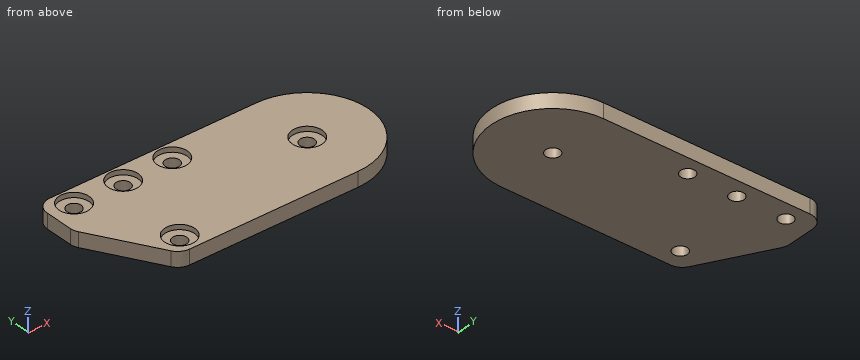
```python
from build123d import *

# Parameters (mm, degrees)
SKETCH_2_R          = 1.45
EXTRUDE_1_DEPTH     = 3
SKETCH_3_R          = 1.45
EXTRUDE_2_DEPTH     = 3
SKETCH_5_R          = 3.05
CUT_EXTRUDE_1_DEPTH = 1
EXTRUDE_3_DEPTH     = 3
SKETCH_7_R          = 3.05
CUT_EXTRUDE_4_DEPTH = 1
FILLET_1_R          = 3
SKETCH_10_R         = 3.05
CUT_EXTRUDE_6_DEPTH = 1


with BuildPart() as part:
    # 草图2 → 凸台-拉伸1 (new body)
    with BuildSketch(Plane.XY):
        with BuildLine():
            Line((-10, -7), (-10, -16.423561614))
            Line((-10, -16.423561614), (30.724748208, -31.24615776))
            ThreePointArc((30.724748208, -31.24615776), (47.310096913, -21.670602221), (35, -7))
            Line((35, -7), (-10, -7))
        make_face()
        with Locations((35, -19.5)):
            Circle(SKETCH_2_R, mode=Mode.SUBTRACT)
        with Locations((15, -10.5)):
            Circle(SKETCH_2_R, mode=Mode.SUBTRACT)
        with Locations((5, -10.5)):
            Circle(SKETCH_2_R, mode=Mode.SUBTRACT)
        with Locations((-5, -10.5)):
            Circle(SKETCH_2_R, mode=Mode.SUBTRACT)
    extrude(amount=EXTRUDE_1_DEPTH)

    # 草图3 → 凸台-拉伸2 (add)
    with BuildSketch(Plane.XY.offset(3)):
        Polygon((-10, -16.423561614), (32.795912741, -32), (-1.006939105, -32), align=None)
        with Locations((2, -28)):
            Circle(SKETCH_3_R, mode=Mode.SUBTRACT)
    extrude(amount=-EXTRUDE_2_DEPTH)

    # 草图5 → 切除-拉伸1 (cut)
    with BuildSketch(Plane.XY.offset(3)):
        with Locations((-5, -10.5)):
            Circle(SKETCH_5_R)
        with Locations((5, -10.5)):
            Circle(SKETCH_5_R)
        with Locations((15, -10.5)):
            Circle(SKETCH_5_R)
    extrude(amount=-CUT_EXTRUDE_1_DEPTH, mode=Mode.SUBTRACT)

    # 草图8 → 凸台-拉伸3 (add)
    with BuildSketch(Plane.XY.offset(3)):
        Polygon((32.795912741, -32), (35, -32), (30.724748208, -31.24615776), align=None)
    extrude(amount=-EXTRUDE_3_DEPTH)

    # 草图7 → 切除-拉伸4 (cut)
    with BuildSketch(Plane.XY.offset(3)):
        with Locations((2, -28)):
            Circle(SKETCH_7_R)
    extrude(amount=-CUT_EXTRUDE_4_DEPTH, mode=Mode.SUBTRACT)

    # 圆角1
    fillet_1_edges = [part.edges().sort_by_distance(p)[0] for p in [
        (-1.006939105, -32, 1.5),
        (-10, -16.423561614, 1.5),
        (-10, -7, 1.5),
    ]]
    fillet(fillet_1_edges, radius=FILLET_1_R)

    # 草图10 → 切除-拉伸6 (cut)
    with BuildSketch(Plane.XY.offset(3)):
        with Locations((35, -19.5)):
            Circle(SKETCH_10_R)
    extrude(amount=-CUT_EXTRUDE_6_DEPTH, mode=Mode.SUBTRACT)


solid = part.part
```
Read the model definition and answer for the solid it produces. Units are mm, in the model's axes. Coordinates: 2 decimals unless noted, no trailing zeros. Write each loop counter-clockwise with the first axis right and the second up, starting at its lowest first coordinate (ties: lowest second). Pieces come first, ordered by that corner, then holes. Notation, with made-up numbers: (77.5, 42.25) -> (102.5, 42.25) arc R31 cw to (102.5, 80.25) -> close; hole circle Ø1 at (45.5, 57). An arc over 180 degrees is marked (long way). Answer as a JSON object with one key per item and string values.
Q1. The part is cut by section A-A on x = 15. Give the vertices of the cut face in (y, z), then the cut area to 3 significant figures.
The answers:
{"outline": "(-32, 0) -> (-11.95, 0) -> (-11.95, 2) -> (-13.55, 2) -> (-13.55, 3) -> (-32, 3) -> close; (-9.05, 0) -> (-7, 0) -> (-7, 3) -> (-7.45, 3) -> (-7.45, 2) -> (-9.05, 2) -> close", "area": "63.1 mm2"}
Q2. The part is cut by section B-B on z = 1.15. Give the vertices of the cut face in (x, y).
The answers:
{"outline": "(-10, -15.62) arc R3 ccw to (-9.6, -17.12) -> (-1.87, -30.5) arc R3 ccw to (0.73, -32) -> (35, -32) arc R12.5 ccw to (35, -7) -> (-7, -7) arc R3 ccw to (-10, -10) -> close; hole circle Ø2.9 at (-5, -10.5); hole circle Ø2.9 at (2, -28); hole circle Ø2.9 at (5, -10.5); hole circle Ø2.9 at (15, -10.5); hole circle Ø2.9 at (35, -19.5)"}
Q3. Consider line 1 (Y direction, x = 35, z = 2.7); line 2 (Y direction, x = 35, z = 0.95); line 3 (X direction, y = -10, z = 1). Determine where each line is inside the solid, lowest interval first. Write a range as [from, to].
The answers:
{"line 1": "y = [-32, -22.55], [-16.45, -7]", "line 2": "y = [-32, -20.95], [-18.05, -7]", "line 3": "x = [-10, -6.36], [-3.64, 3.64], [6.36, 13.64], [16.36, 43.12]"}
Q4. Flat-ended cylindrical pins translate along their axes: pin 1 Ø1.8 at (x, y) = (-6, -10.5) entering from +Z; pin 2 Ø3.5 at (x, y) = (15, -10.5) entering from -Z; pin 3 Ø2.5 at (x, y) = (15, -10.5) entering from -Z. Find the tip coordinate at first contact, or state that the pin passes through.
The answers:
{"pin 1": "stops at z = 2", "pin 2": "stops at z = 0", "pin 3": "passes through"}
Q5. The part is cut by section C-C on y = -19.5. Give the vertices of the cut face in (x, z).
The answers:
{"outline": "(-8.22, 0) -> (33.55, 0) -> (33.55, 2) -> (31.95, 2) -> (31.95, 3) -> (-8.22, 3) -> close; (36.45, 0) -> (47.5, 0) -> (47.5, 3) -> (38.05, 3) -> (38.05, 2) -> (36.45, 2) -> close"}
